For this review, take the finished solid that the model builds, in its own axes (mm). A direction names the side the tool comes from. Give positions to 0.01 mm unless a question says otherwise; leave off trailing zeros. Write each loop counter-clockwise with the first axis right and the second up, starting at its lowest first coordinate (ties: lowest second). Pieces come first, ordered by that corner, then holes.
1) We need section A-A on x = 8. Give the boundary of the cut face in (y, z).
2) Wall thickness on line 1 along X through (y, z) = (0.5, -1) (3 decimals); line 2 along Z through (x, y) = (8.5, 0); line 3 along Y through (x, z) = (7.25, 0.5): over which ranges is each line inside the solid? List them lowest first.
3) For P1, Ø0.7, axis at x = -1, z = 0, coming from the -Y side; P2, Ø1, axis at x = 6, z = 2, coming from the -Y side (3 decimals); P3, Ø1, axis at x = 3.5, z = 1, coming from the +Y side, all flat-tipped, find the tip position at first contact; note any pin that passes through.
4) Draft analysis for pull direction Y (two halves, no side actions). For faces 1 (the face through (-0.226, 0, 0)), 2 (the face through (4.59, 1.987, 0.626)), 3 (the face through (0, 2, -2)), state which applies: pulls with the +Y half, pulls with the -Y half, needs draft (parallel to the pull), parting line crosses it, or undercut.
5) Machinability: for faces 4 (the face through (9.525, 0, 0)), 5 (the face through (-1, 1.191, 0)), which of the approach directions +Z, -Z, +X, -X, +Y, -Y give a long, thin tool a straight path to every point of the face, cutting with its end or side? Answer none if there is none.
Autodesk Inventor part; units mm, degrees
ref_plane "screw_XY" through (0, 0, 0) normal (1, 0, 0) x (0, 0, -1)
ref_plane "screw_YZ" through (0, 0, 0) normal (0, 0, -1) x (0, 1, 0)
ref_plane "screw_ZX" through (0, 0, 0) normal (0, 1, 0) x (1, 0, 0)
sketch "Sketch_1" plane through (0, 0, 0) normal (0, 0, 1) x (1, 0, 0)
  line L0 (9.525, 0) -> (-2.2098, 0)
  line L1 (-2.2098, 0) -> (-2.2098, 2.0828)
  arc A0 (-0.2794, 3.9688) -> (-2.2098, 2.0828) centre (1.7151, -0.0037) ccw
  line L2 (-0.2794, 3.9688) -> (0, 3.9688)
  line L3 (0, 3.9688) -> (0, 2.0828)
  line L4 (0, 2.0828) -> (9.0526, 2.0828)
  line L5 (9.0526, 2.0828) -> (9.525, 1.6104)
  line L6 (9.525, 1.6104) -> (9.525, 0)
  line L7 (9.525, 0) -> (-2.2098, 0)
revolve "Revolution1" add sketch "Sketch_1" angle 360 about axis through (9.525, 0, 0) along (1, 0, 0)
thread "Thread1"
sketch "Sketch_3" plane through (-2.2098, 0, 0) normal (1, 0, 0) x (0, 0, -1)
  line L0 (-1.3748, 0) -> (-0.6874, -1.1906)
  line L1 (-0.6874, -1.1906) -> (0.6874, -1.1906)
  line L2 (0.6874, -1.1906) -> (1.3748, 0)
  line L3 (1.3748, 0) -> (0.6874, 1.1906)
  line L4 (0.6874, 1.1906) -> (-0.6874, 1.1906)
  line L5 (-0.6874, 1.1906) -> (-1.3748, 0)
extrude "Extrusion1" cut sketch "Sketch_3" along normal mid plane 3.9675
ref_plane "screw_XY" through (0, 0, 0) normal (1, 0, 0) x (0, 0, -1)
ref_plane "screw_YZ" through (0, 0, 0) normal (0, 0, -1) x (0, 1, 0)
ref_plane "screw_ZX" through (0, 0, 0) normal (0, 1, 0) x (1, 0, 0)
ref_plane "to_nut_XY" through (9.525, 0, 0) normal (1, 0, 0) x (0, 0, -1)
ref_plane "to_nut_YZ" through (9.525, 0, 0) normal (0, 0, -1) x (0, 1, 0)
ref_plane "to_nut_ZX" through (9.525, 0, 0) normal (0, 1, 0) x (1, 0, 0)
properties part number "3005"
Results list:
1. outline: circle Ø4.17 at (0, 0)
2. line 1: x = -0.226 to 9.525
2. line 2: z = -2.08 to 2.08
2. line 3: y = -2.02 to 2.02
3. P1: stops at y = -3.76
3. P2: stops at y = -1.445
3. P3: stops at y = 2.02
4. face 1: undercut
4. face 2: parting line crosses it
4. face 3: needs draft
5. face 4: +Z, -Z, +X, +Y, -Y
5. face 5: -X
